from build123d import *

# Parameters (mm, degrees)
F0_R     = 3.175
F0_R_2   = 1.5875
F1_DEPTH = 25.4
F2_DEPTH = 25.4
F3_DEPTH = 25.4


with BuildPart() as f1:
    # F0 (on Front) → F1 (new body)
    with BuildSketch(Plane.XZ):
        with BuildLine():
            ThreePointArc((0.34017864, 9.5189234419), (0.170116454, 9.5234807393), (0, 9.525))
            ThreePointArc((0, 9.525), (-7.044647886, 6.4108159514), (-9.4828222655, -0.8953808583))
            ThreePointArc((-9.4828222655, -0.8953808583), (-6.4108159514, -7.044647886), (0, -9.525))
            Line((0, -9.525), (0.6773435479, -9.500885786))
            ThreePointArc((0.6773435479, -9.500885786), (6.9705567315, -6.4912990883), (9.525, 0))
            ThreePointArc((9.525, 0), (6.8544083095, 6.6138273131), (0.34017864, 9.5189234419))
        make_face()
        with BuildLine():
            ThreePointArc((3.175, 0), (-2.2450640303, -2.2450640303), (0, 3.175))
            ThreePointArc((0, 3.175), (2.2450640303, 2.2450640303), (3.175, 0))
        make_face(mode=Mode.SUBTRACT)
        with BuildLine():
            ThreePointArc((-9.4828222655, -0.8953808583), (-7.044647886, 6.4108159514), (0, 9.525))
            Line((0, 9.525), (0, 9.5310804347))
            Line((0, 9.5310804347), (0, 47.625))
            ThreePointArc((0, 47.625), (-9.3346028611, 50.6594075516), (-15.1007031189, 58.6026139305))
            Line((-15.1007031189, 58.6026139305), (-9.4828222655, -0.8953808583))
        make_face()
        with BuildLine():
            Line((0, 47.625), (0, 9.5310804347))
            Line((0, 9.5310804347), (0.34017864, 9.5189234419))
            Line((0.34017864, 9.5189234419), (10.4321012974, 9.1582675492))
            Line((10.4321012974, 9.1582675492), (15.1007031189, 58.6026139305))
            ThreePointArc((15.1007031189, 58.6026139305), (9.3346028611, 50.6594075516), (0, 47.625))
        make_face()
        with BuildLine():
            Line((10.4321012974, 9.1582675492), (0.34017864, 9.5189234419))
            ThreePointArc((0.34017864, 9.5189234419), (6.8544083095, 6.6138273131), (9.525, 0))
            ThreePointArc((9.525, 0), (6.9705567315, -6.4912990883), (0.6773435479, -9.500885786))
            Line((0.6773435479, -9.500885786), (44.7324052746, -7.9324746146))
            ThreePointArc((44.7324052746, -7.9324746146), (36.5125000183, 0.0005387766), (44.7334821429, 7.9324362036))
            Line((44.7334821429, 7.9324362036), (10.4321012974, 9.1582675492))
        make_face()
        with BuildLine():
            ThreePointArc((-15.1007031189, 58.6026139305), (-9.3346028611, 50.6594075516), (0, 47.625))
            Line((0, 47.625), (0, 60.325))
            ThreePointArc((0, 60.325), (-3.175, 63.5), (0, 66.675))
            Line((0, 66.675), (0, 79.375))
            ThreePointArc((0, 79.375), (-10.5003255158, 75.40625), (-15.7504882737, 65.484375))
            Line((-15.7504882737, 65.484375), (-15.1007031189, 58.6026139305))
        make_face()
        with BuildLine():
            Line((0, 60.325), (0, 47.625))
            ThreePointArc((0, 47.625), (9.3346028611, 50.6594075516), (15.1007031189, 58.6026139305))
            Line((15.1007031189, 58.6026139305), (15.7504882737, 65.484375))
            ThreePointArc((15.7504882737, 65.484375), (10.5003255158, 75.40625), (0, 79.375))
            Line((0, 79.375), (0, 66.675))
            ThreePointArc((0, 66.675), (2.2450640303, 65.7450640303), (3.175, 63.5))
            ThreePointArc((3.175, 63.5), (2.2450640303, 61.2549359697), (0, 60.325))
        make_face()
        with BuildLine():
            Line((0.6773435479, -9.500885786), (0, -9.525))
            ThreePointArc((0, -9.525), (0.3388863295, -9.5189695375), (0.6773435479, -9.500885786))
        make_face()
        with BuildLine():
            ThreePointArc((-15.7504882737, 65.484375), (-15.8047037758, 62.0076985695), (-15.1007031189, 58.6026139305))
            Line((-15.1007031189, 58.6026139305), (-15.7504882737, 65.484375))
        make_face()
        with BuildLine():
            Line((15.7504882737, 65.484375), (15.1007031189, 58.6026139305))
            ThreePointArc((15.1007031189, 58.6026139305), (15.6802309775, 61.020890988), (15.875, 63.5))
            ThreePointArc((15.875, 63.5), (15.8438414904, 64.4941387366), (15.7504882737, 65.484375))
        make_face()
        with BuildLine():
            ThreePointArc((52.3875, 0), (50.1620069047, 5.5115227815), (44.7334821429, 7.9324362036))
            ThreePointArc((44.7334821429, 7.9324362036), (36.5125000183, 0.0005387766), (44.7324052746, -7.9324746146))
            ThreePointArc((44.7324052746, -7.9324746146), (50.1616327839, -5.5119104847), (52.3875, 0))
        make_face()
        with Locations((44.45, 0)):
            Circle(F0_R, mode=Mode.SUBTRACT)
        with BuildLine():
            Line((-9.4502929642, 115.490625), (-15.7504882737, 65.484375))
            ThreePointArc((-15.7504882737, 65.484375), (-10.5003255158, 75.40625), (0, 79.375))
            Line((0, 79.375), (0, 104.775))
            ThreePointArc((0, 104.775), (-7.14375, 107.9998046905), (-9.4502929642, 115.490625))
        make_face()
        with Locations((-3.5204379819, 97.8255793452)):
            Circle(F0_R_2, mode=Mode.SUBTRACT)
        with BuildLine():
            ThreePointArc((0, 79.375), (10.5003255158, 75.40625), (15.7504882737, 65.484375))
            Line((15.7504882737, 65.484375), (9.4502929642, 115.490625))
            ThreePointArc((9.4502929642, 115.490625), (9.5063048942, 114.896483242), (9.525, 114.3))
            ThreePointArc((9.525, 114.3), (6.7351920908, 107.5648079092), (0, 104.775))
            Line((0, 104.775), (0, 79.375))
        make_face()
        with BuildLine():
            ThreePointArc((9.4502929642, 115.490625), (0, 123.825), (-9.4502929642, 115.490625))
            ThreePointArc((-9.4502929642, 115.490625), (-7.14375, 107.9998046905), (0, 104.775))
            ThreePointArc((0, 104.775), (6.7351920908, 107.5648079092), (9.525, 114.3))
            ThreePointArc((9.525, 114.3), (9.5063048942, 114.896483242), (9.4502929642, 115.490625))
        make_face()
        with BuildLine():
            ThreePointArc((3.175, 114.3), (2.2450640303, 112.0549359697), (0, 111.125))
            ThreePointArc((0, 111.125), (-2.2450640303, 116.5450640303), (3.175, 114.3))
        make_face(mode=Mode.SUBTRACT)
    extrude(amount=F1_DEPTH)

    # F2 (add): a face of the model
    f2_faces = [f1.faces().sort_by_distance(p)[0] for p in [
        (5.1424381461, -25.4, 47.1936001946),
    ]]
    extrude(f2_faces, amount=F2_DEPTH)

    # F3 (add): a face of the model
    f3_faces = [f1.faces().sort_by_distance(p)[0] for p in [
        (5.1424381461, -50.8, 47.1936001946),
    ]]
    extrude(f3_faces, amount=F3_DEPTH)


solid = f1.part
Input: part model. Units: mm. Frame: model coordinates. A direction names the side the tool comes from. Give positions to 0.01 mm unless a question says otherwise; leave off trailing zeros. Write each loop counter-clockwise with the first axis right and the second up, starting at its lowest first coordinate (ties: lowest second). Pieces come first, ordered by that corner, then holes.
Q1. First-contact query: P1, Ø2, axis at y = -18, z = 55, coming from the +X side; P2, Ø4, axis at x = 34, y = -50.5, coming from the +Z side; P3, Ø5, axis at y = -21.5, z = 87, coming from the -X side. Flat tips, straight axial feed; report the tip coordinate or a pass-through.
Q2. Section C-C, the plane x = 27. Output: boundary loops of the cut face in (y, z), plus the area to 3 significant figures.
Q3. Section A-A, the plane z = 63.5. Output: boundary loops of the cut face in (x, y) (3 decimals).
Q4. Pull-direction query (X, two-part tool) for faces 3 (the face through (3, 0, 43)), 4 (the face through (-12.556, -37.567, 90.838)), 5 (the face through (3.03, -37.57, 62.55)), 6 (the face through (52.386, -37.567, -0.171)); classes: pulls with the +X half, pulls with the -X half, needs draft (parallel to the pull), parting line crosses it, or undercut.
Q5. Section D-D, the plane z = 80. Output: boundary loops of the cut face in (x, y).
Q6. Material intervals for probe 1 along X at (y, z) = (-35, 62); probe 2 along X at (y, z) = (-25.5, 114.3) (3 decimals); probe 3 along X at (y, z) = (-71, 89), sorted ascending.
Q7. Set-up query: faces 1 (the face through (12.734, -37.567, 33.534)), 2 (the face through (12.644, -37.567, 90.137)). Return all of +Z, -Z, +X, -X, +Y, -Y with unobstructed straight access to the full face (end or side cutting, diameter ignored); none if empty.
Filled in:
1. P1: stops at x = 14.85
1. P2: stops at z = 8.39
1. P3: stops at x = -13.35
2. outline: (-76.2, -8.56) - (0, -8.56) - (0, 8.57) - (-76.2, 8.57) - close
2. area: 1,310 mm2
3. outline: (-15.875, -76.2) - (-3.175, -76.2) - (-3.175, 0) - (-15.875, 0) - close; (3.175, -76.2) - (15.875, -76.2) - (15.875, 0) - (3.175, 0) - close
4. face 3: needs draft
4. face 4: pulls with the -X half
4. face 5: undercut
4. face 6: pulls with the +X half
5. outline: (-13.92, -76.2) - (13.92, -76.2) - (13.92, 0) - (-13.92, 0) - close
6. probe 1: x = -15.8 to -2.8, 2.8 to 15.8
6. probe 2: x = -9.6 to -3.175, 3.175 to 9.6
6. probe 3: x = -12.79 to 12.79
7. face 1: +X, +Y, -Y
7. face 2: +Z, +X, +Y, -Y
